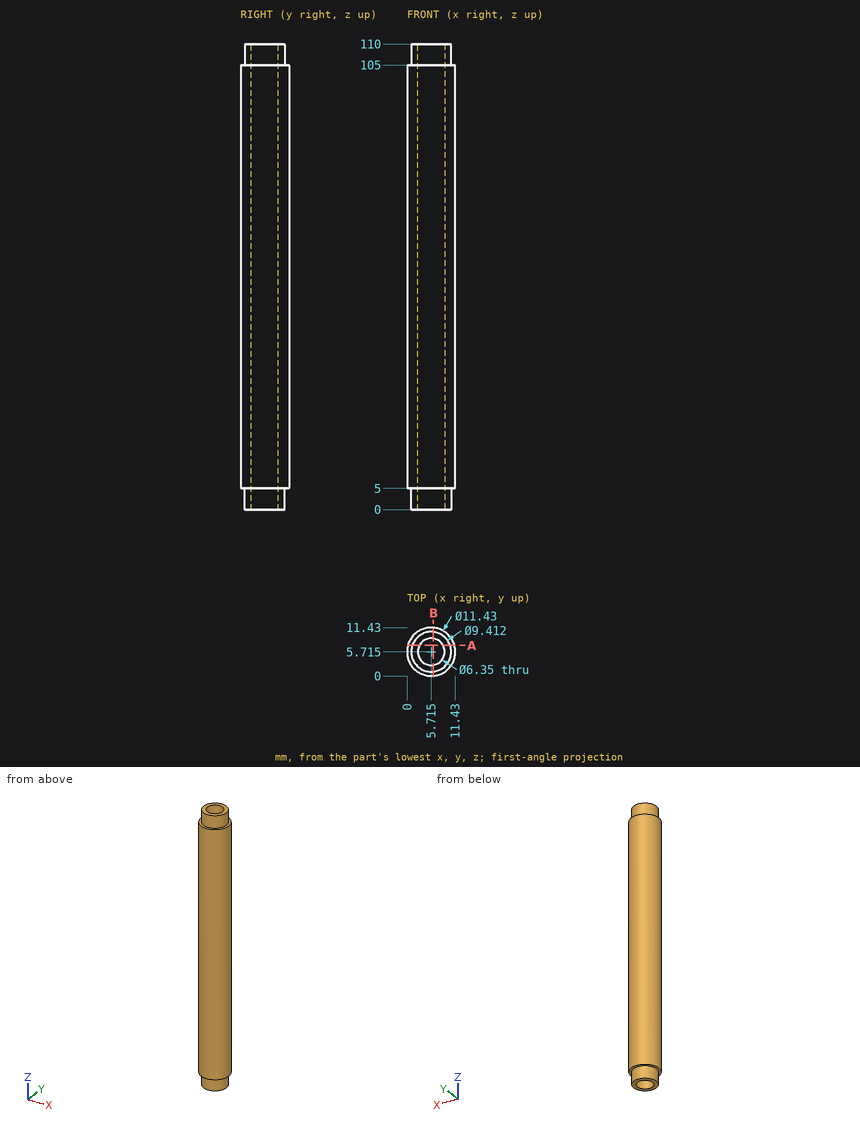
Design review of the part shown in the three views and the two pictorial views. Dimensions are in mm from the part's minimum x, y and z. Coordinates: 2 decimals unless noted, no trailing zeros. Loops run counter-clockwise (first coordinate to the right, second up) from the corner with the lowest first, then second, coordinate; pieces in that order, holes last.
Q1. To check wall thickness, follow line 1 (X direction, y = 5.5, z = 61.5) (1 decimal); line 2 (X direction, y = 6, z = 10); line 3 (Y direction, x = 6.75, z = 85.5) (1 decimal). State the ranges of each line that lie inside material, in increasing order.
Reported:
line 1: x = 0 to 2.5, 8.9 to 11.4
line 2: x = 0.01 to 2.55, 8.88 to 11.42
line 3: y = 0.1 to 2.7, 8.7 to 11.3
Q2. For pin 1 (2 mm diameter, centred on x = 9.5, y = 3, fed in from -Z); pin 2 (1 mm diameter, centred on x = 8, z = 48, fed in from +Y) (1 decimal), all flat-tipped, find the tip position at first contact; note any pin that passes through.
Reported:
pin 1: stops at z = 0
pin 2: stops at y = 11.1
Q3. We need section A-A on y = 7.25. State the section outline as (x, z) points (1 decimal).
Reported:
outline: (0.2, 5) - (1.3, 5) - (1.3, 0) - (2.9, 0) - (2.9, 110) - (1.3, 110) - (1.3, 105) - (0.2, 105) - close; (8.5, 0) - (10.2, 0) - (10.2, 5) - (11.2, 5) - (11.2, 105) - (10.2, 105) - (10.2, 110) - (8.5, 110) - close
Q4. We need section B-B on x = 6.25. State the section outline as (y, z) points (1 decimal).
Reported:
outline: (0, 5) - (1, 5) - (1, 0) - (2.6, 0) - (2.6, 110) - (1, 110) - (1, 105) - (0, 105) - close; (8.8, 0) - (10.4, 0) - (10.4, 5) - (11.4, 5) - (11.4, 105) - (10.4, 105) - (10.4, 110) - (8.8, 110) - close
